Check sheet for the drawn part. Datum: minimum x, y, z corner. Units: mm. A direction names the side the tool comes from. Round coordinates to 2 decimals unless told otherwise and drop trailing zeros. Order: outer loops, then holes, each group sorted by start corner. A loop starts at its lowest first (then second) coordinate and runs counter-clockwise, first axis right, second up. Notation, with made-up numbers: (-36, 28.25) - (-7, 28.25) arc R11 cw to (-7, 40.25) - close; hole circle Ø3 at (-6.5, 79). An arc over 180 degrees is marked (long way). Write each question's results on one line, items separated by ' | '.
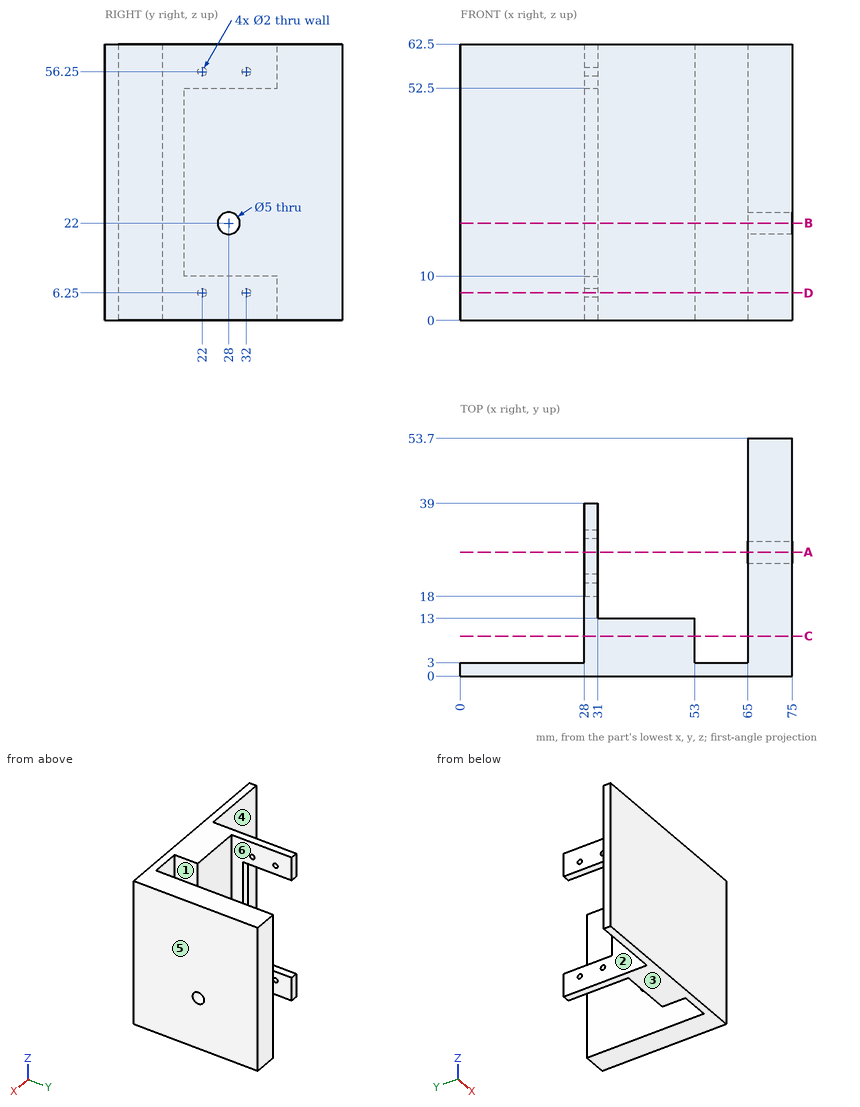
(1) Section check C-C (y = 9). Record the cut outline in (x, z), then the cut area to 3 significant figures.
Answers follow:
outline: (28, 0) - (53, 0) - (53, 62.5) - (28, 62.5) - close; (65, 0) - (75, 0) - (75, 62.5) - (65, 62.5) - close | area: 2,190 mm²
(2) Section check D-D (z = 6.25). Record the cut outline in (x, y).
Answers follow:
outline: (0, 0) - (75, 0) - (75, 53.7) - (65, 53.7) - (65, 3) - (53, 3) - (53, 13) - (31, 13) - (31, 21) - (28, 21) - (28, 3) - (0, 3) - close; (28, 23) - (31, 23) - (31, 31) - (28, 31) - close; (28, 33) - (31, 33) - (31, 39) - (28, 39) - close
(3) Section check A-A (y = 28). Record the cut outline in (x, z), then the cut area to 3 significant figures.
Answers follow:
outline: (28, 0) - (31, 0) - (31, 10) - (28, 10) - close; (28, 52.5) - (31, 52.5) - (31, 62.5) - (28, 62.5) - close; (65, 0) - (75, 0) - (75, 19.5) - (65, 19.5) - close; (65, 24.5) - (75, 24.5) - (75, 62.5) - (65, 62.5) - close | area: 635 mm²
(4) Section check B-B (z = 22). Record the cut outline in (x, y), then the cut area to 3 significant figures.
Answers follow:
outline: (0, 0) - (75, 0) - (75, 25.5) - (65, 25.5) - (65, 3) - (53, 3) - (53, 13) - (31, 13) - (31, 18) - (28, 18) - (28, 3) - (0, 3) - close; (65, 30.5) - (75, 30.5) - (75, 53.7) - (65, 53.7) - close | area: 947 mm²
(5) Depth check by flat-ended pin: pin 1 Ø2.5 at (y, z) = (22, 56.25) entering from -X; pin 2 Ø3 at (x, z) = (63, 10) entering from +Y; pin 3 Ø3.5 at (x, z) = (29.5, 22) entering from +Y. Enter the tip coordinate at first touch or a pass-through.
Answers follow:
pin 1: x = 28 | pin 2: y = 3 | pin 3: y = 18
(6) Draft check along X on the marked faces 1, 2 and 3. Enter one of: released by +X, released by -X, zero draft, split by the parting line, or undercut.
Answers follow:
face 1: undercut | face 2: released by -X | face 3: zero draft
(7) Access from +Z, -Z, +X, -X, +Y, -Y to the whole of each face (thin tool, end or side, straight path). Record for the marked faces 4, 5 and 6.
Answers follow:
face 4: +Z, -Z, -X, +Y | face 5: +Z, -Z, +X, +Y, -Y | face 6: +Z, -Z, +Y
(8) Material ranges on line 1 (Y direction, x = 29, z = 56.25); line 2 (X direction, y = 17.5, z = 36.5); line 3 (Y direction, x = 68, z = 22), recorded low to high.
Answers follow:
line 1: 0 to 21, 23 to 31, 33 to 39 | line 2: 28 to 31, 65 to 75 | line 3: 0 to 25.5, 30.5 to 53.7
